Geometry check sheet. Reference: the model listing, model coordinates, mm. Face numbers are marked on the shaded views. Give positions to 0.01 mm unless a question says otherwise; leave off trailing zeros. Order: outer loops, then holes, each group sorted by start corner. A loop starts at its lowest first (then second) coordinate and runs counter-clockwise, first axis right, second up. Notation, with made-up numbers: M 24,-13 L 77,-13 A28 ccw 77,8 Z; hole C -34.75,54 d3. An arc over 180 degrees is marked long. Use CSV: the item, a comma, the result in double quotes. Start each with the question number.
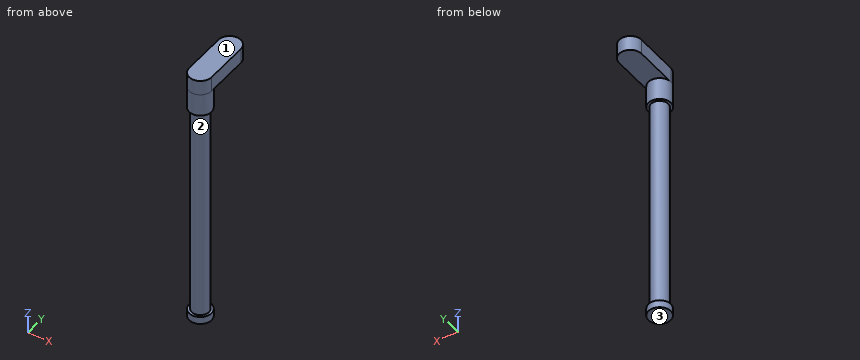
from build123d import *

# Parameters (mm, degrees)
F0_R     = 2.921
F1_DEPTH = 73.66
F2_R     = 3.81
F2_R_2   = 2.921
F3_DEPTH = 2.54
F4_R     = 3.81
F5_DEPTH = 7.62
F7_DEPTH = 5.08


with BuildPart() as f1:
    # F0 (on Top) → F1 (new body)
    with BuildSketch(Plane.XY):
        Circle(F0_R)
    extrude(amount=F1_DEPTH)

    # F2 (on face) → F3 (join)
    with BuildSketch(Plane(origin=(0, 0, 0), x_dir=(1, 0, 0), z_dir=(0, 0, -1))):
        Circle(F2_R)
        Circle(F2_R_2, mode=Mode.SUBTRACT)
        Circle(F2_R_2)
    extrude(amount=F3_DEPTH)

    # F4 (on face) → F5 (join)
    with BuildSketch(Plane.XY.offset(73.66)):
        Circle(F4_R)
    extrude(amount=F5_DEPTH)

    # F6 (on face) → F7 (join)
    with BuildSketch(Plane.XY.offset(81.28)):
        with BuildLine():
            ThreePointArc((-3.81, 0), (0, 3.81), (3.81, 0))
            Line((3.81, 0), (3.81, 15.24))
            ThreePointArc((3.81, 15.24), (0, 11.43), (-3.81, 15.24))
            Line((-3.81, 15.24), (-3.81, 0))
        make_face()
        with BuildLine():
            Line((-3.81, 0), (3.81, 0))
            ThreePointArc((3.81, 0), (0, 3.81), (-3.81, 0))
        make_face()
        with BuildLine():
            ThreePointArc((-3.81, 0), (0, -3.81), (3.81, 0))
            Line((3.81, 0), (-3.81, 0))
        make_face()
        with BuildLine():
            Line((-3.81, 15.24), (3.81, 15.24))
            ThreePointArc((3.81, 15.24), (0, 19.05), (-3.81, 15.24))
        make_face()
        with BuildLine():
            ThreePointArc((-3.81, 15.24), (0, 11.43), (3.81, 15.24))
            Line((3.81, 15.24), (-3.81, 15.24))
        make_face()
    extrude(amount=F7_DEPTH)


solid = f1.part
(1) Draft check along Z on the marked faces 1, 2 and 3. Enter one of: +Z half, -Z half, draft (parallel to the pull), parting line (faces both ways), or undercut.
(2) Sectioned sample at B-B on y = 8.75. Record the cut outline in (x, z).
(3) Sectioned sample at C-C on z = 33.5. Record the cut outline in (x, y), then the cut area to 3 significant figures.
(4) Thickness scan on line 1 (Z direction, x = -0.5, y = 15); line 2 (Y direction, x = 1.75, z = 19); line 3 (Y direction, x = -2.5, z = 30). Record the ranges inside material, lowest first.
(5) Go/stop test with flat-tipped pins: P1, Ø2.5, axis at x = 1, y = 8.5, coming from the -Z side; P2, Ø10, axis at y = 2.5, z = 67.5, coming from the -X side; P3, Ø1.5, axis at x = 2, z = 59.5, coming from the +Y side. Record where each tip stops, or that it passes through.
(6) Sectioned sample at D-D on z = 77. Record the cut outline in (x, y).
(7) Sectioned sample at A-A on x = 0. Record the cut outline in (y, z), then the cut area to 3 significant figures.
Responses:
1,face 1,"+Z half"
1,face 2,"undercut"
1,face 3,"-Z half"
2,outline,"M -3.81,81.28 L 3.81,81.28 L 3.81,86.36 L -3.81,86.36 Z"
3,outline,"C 0,0 d5.84"
3,area,"26.8 mm2"
4,line 1,"81.28 to 86.36"
4,line 2,"-2.34 to 2.34"
4,line 3,"-1.51 to 1.51"
5,P1,"z = 81.28"
5,P2,"x = -2.92"
5,P3,"y = 2.64"
6,outline,"C 0,0 d7.62"
7,outline,"M -3.81,-2.54 L 3.81,-2.54 L 3.81,0 L 2.92,0 L 2.92,73.66 L 3.81,73.66 L 3.81,81.28 L 19.05,81.28 L 19.05,86.36 L -3.81,86.36 L -3.81,73.66 L -2.92,73.66 L -2.92,0 L -3.81,0 Z"
7,area,"624 mm2"
